Read the model definition and answer for the solid it produces. Units are mm, in the model's axes. Face numbers are marked on the shaded views. A direction names the side the tool comes from. Coordinates: 2 decimals unless noted, no trailing zeros. Loops run counter-clockwise (first coordinate to the right, second up) from the corner with the lowest first, then second, coordinate; pieces in that order, holes last. Notation, with made-up numbers: (37.25, 80) -> (43.25, 80) arc R32 ccw to (43.25, 110) -> close; hole circle Ø3 at (12.5, 22). An arc over 180 degrees is marked (long way). Answer as a JSON object with one key per item and string values. Group by question number.
Q1. The part is cut by section A-A on x = 17. Write down the section's boundary in (y, z).
Q2. The part is cut by section D-D on z = 3. Write down the section's boundary in (x, y), and give its area (3 significant figures).
Q3. Straight lines are drawn through the part: line 1 along X through (y, z) = (1.75, -10); line 2 along X through (y, z) = (3.7, 12.5); line 3 along Z through (x, y) = (16.5, 4.6). For each, find the intervals that lie inside material, in ascending order. Write a range as [from, to].
Q4. Each of these flat-tipped pins is pushed along its axis until it touches: P1, Ø12, axis at x = -4.5, z = 4.5, coming from the -Y side; P2, Ø0.7, axis at x = 9.5, z = 13, coming from the +Y side; P3, Ø0.9, axis at y = 4, z = -4, coming from the +X side. Where does it stop, or does it pass through?
Q5. The part is cut by section C-C on x = 10. Write down the section's boundary in (y, z).
Q6. The part is cut by section B-B on z = -10. Write down the section's boundary in (x, y).
Q7. For the marked faces 1 and 2, determine the directions among +Z, -Z, +X, -X, +Y, -Y from which every point of the face is accessible in a straight line to the end or side of a thin tool.
Q8. Determine the mould class of the marked faces 3, 4 and 5 for opening direction Z: released by +Z, released by -Z, zero draft, split by the parting line, or undercut.
from build123d import *

# Parameters (mm, degrees)
SKETCH1_W           = 44
SKETCH1_H           = 30
BOSS_EXTRUDE1_DEPTH = 5
SKETCH2_W           = 8
SKETCH2_H           = 30
BOSS_EXTRUDE2_DEPTH = 1
SKETCH3_R           = 1.55
CUT_EXTRUDE1_DEPTH  = 28.294688128
CUT_EXTRUDE2_DEPTH  = 3
SKETCH7_R           = 1.1
CUT_EXTRUDE4_DEPTH  = 2
SKETCH5_R           = 0.889
CUT_EXTRUDE5_DEPTH  = 27.795522014
SKETCH6_R           = 0.889
CUT_EXTRUDE6_DEPTH  = 28.294688128
CHAMFER2_SIZE       = 3
CHAMFER2_SIZE_2     = 0.39


with BuildPart() as part:
    # Sketch1 → Boss-Extrude1 (new body)
    with BuildSketch(Plane(origin=(0, 0, 0), x_dir=(1, 0, 0), z_dir=(0, 1, 0))):
        Rectangle(SKETCH1_W, SKETCH1_H)
    extrude(amount=BOSS_EXTRUDE1_DEPTH)

    # Sketch2 → Boss-Extrude2 (add)
    with BuildSketch(Plane.XZ):
        with Locations((-18, 0)):
            Rectangle(SKETCH2_W, SKETCH2_H)
    extrude(amount=BOSS_EXTRUDE2_DEPTH)

    # Sketch3 → Cut-Extrude1 (cut, through all)
    with BuildSketch(Plane(origin=(0, 5, 0), x_dir=(1, 0, 0), z_dir=(0, 1, 0))):
        with Locations(Location((-6, 10, 0), (0, 0, 270))):
            Circle(SKETCH3_R)
    extrude(amount=-CUT_EXTRUDE1_DEPTH, mode=Mode.SUBTRACT)

    # Sketch4 → Cut-Extrude2 (cut)
    with BuildSketch(Plane(origin=(0, 5, 0), x_dir=(1, 0, 0), z_dir=(0, 1, 0))):
        Polygon((22, -10), (-20, -10), (-20, -4.75), (-22, -4.75), (-22, 1.25), (-20, 1.25), (-20, 5), (22, 5), align=None)
    extrude(amount=-CUT_EXTRUDE2_DEPTH, mode=Mode.SUBTRACT)

    # Sketch7 → Cut-Extrude4 (cut)
    with BuildSketch(Plane(origin=(0, 5, 0), x_dir=(1, 0, 0), z_dir=(0, 1, 0))):
        with Locations(Location((-19, 12, 0), (0, 0, 270))):
            Circle(SKETCH7_R)
        with Locations(Location((10, -12.5, 0), (0, 0, 270))):
            Circle(SKETCH7_R)
    extrude(amount=-CUT_EXTRUDE4_DEPTH, mode=Mode.SUBTRACT)

    # Sketch5 → Cut-Extrude5 (cut, through all)
    with BuildSketch(Plane(origin=(0, 2, 0), x_dir=(1, 0, 0), z_dir=(0, 1, 0))):
        with Locations(Location((-17.14, -7.14, 0), (0, 0, 270))):
            Circle(SKETCH5_R)
    extrude(amount=-CUT_EXTRUDE5_DEPTH, mode=Mode.SUBTRACT)

    # Sketch6 → Cut-Extrude6 (cut, through all)
    with BuildSketch(Plane(origin=(0, 5, 0), x_dir=(1, 0, 0), z_dir=(0, 1, 0))):
        with Locations(Location((17, 10, 0), (0, 0, 270))):
            Circle(SKETCH6_R)
    extrude(amount=-CUT_EXTRUDE6_DEPTH, mode=Mode.SUBTRACT)

    # Chamfer2
    # the kernel refuses this chamfer: 3, 0.39 mm, written as the material it adds along each edge
    with BuildSketch(Plane(origin=(-20, 2, -5), x_dir=(0, 0.9999877000722414, -0.004959808890380354), z_dir=(1, 0, 0))) as chamfer2_piece_1_section:
        Polygon((CHAMFER2_SIZE * 0.999987700072, CHAMFER2_SIZE * 0.00495980889038), (-CHAMFER2_SIZE_2 * 0.00495980889038, CHAMFER2_SIZE_2 * 0.999987700072), (0, 0), align=None)
    chamfer2_piece_1 = extrude(amount=42, mode=Mode.PRIVATE)
    chamfer2_piece_1 = split(chamfer2_piece_1, bisect_by=Plane(origin=(1, 5, -4.903199608), z_dir=(0, -1, 0)), keep=Keep.TOP, mode=Mode.PRIVATE)
    add(chamfer2_piece_1)


solid = part.part
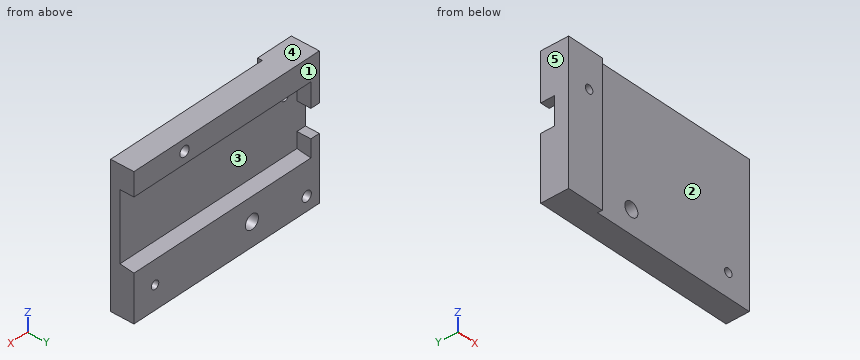
Final values:
{
 "1": {"outline": "(0, -15) -> (5, -15) -> (5, -10.89) -> (0, -10.89) -> close; (0, -9.11) -> (5, -9.11) -> (5, -5) -> (2, -4.61) -> (2, 10) -> (5, 10) -> (5, 15) -> (0, 15) -> close"},
 "2": {"outline": "(-22, -1) -> (-14, -1) -> (-14, 0) -> (22, 0) -> (22, 2) -> (-22, 2) -> close", "area": "96.0 mm2"},
 "3": {"line 1": "x = [-22, -7.55], [-4.45, 16.11], [17.89, 22]", "line 2": "x = [-22, 8.9], [11.1, 22]", "line 3": "z = [-15, -10.74], [-9.26, -4.95], [10, 15]"},
 "4": {"P1": "stops at y = 0", "P2": "stops at y = 3", "P3": "stops at x = -20"},
 "5": {"outline": "(0, -15) -> (5, -15) -> (5, -5) -> (2, -4.61) -> (2, 10) -> (5, 10) -> (5, 11.4) -> (3, 11.4) -> (3, 13.6) -> (5, 13.6) -> (5, 15) -> (0, 15) -> close"},
 "6": {"outline": "(-22, -1) -> (-14, -1) -> (-14, 0) -> (-7.55, 0) -> (-7.55, 5) -> (-22, 5) -> close; (-4.45, 0) -> (16.11, 0) -> (16.11, 5) -> (-4.45, 5) -> close; (17.89, 0) -> (22, 0) -> (22, 5) -> (17.89, 5) -> close"},
 "7": {"face 1": "+Z, -Z, +X, -X, +Y", "face 2": "+Z, -Z, +X, -Y"},
 "8": {"face 3": "undercut", "face 4": "released by +Z", "face 5": "zero draft"}
}
